Build history of the part. All positions in model axes, mm. Face numbers are marked on the shaded views. A direction names the side the tool comes from. Round coordinates to 2 decimals unless told otherwise and drop trailing zeros. Write each loop counter-clockwise with the first axis right and the second up, starting at its lowest first coordinate (ties: lowest second). Pieces come first, ordered by that corner, then holes.
1) Saw through at C-C (y = 7). Write the cut outline in (x, z), plus the area to 3 significant figures.
2) Which spindle directions (+Z, -Z, +X, -X, +Y, -Y) get a long thin tool onto all of the face, cutting with end or side? Do the marked faces 4, 5 and 6. Say none if no direction does.
3) Pull direction X, two halves, no side cores. Call the marked faces 1, 2 and 3: +X half, -X half, draft (parallel to the pull), parting line (faces both ways), or undercut.
4) Saw through at B-B (z = 2.5). Write the cut outline in (x, y), plus the area to 3 significant figures.
5) Saw through at A-A (y = -44). Write the cut outline in (x, z), plus the area to 3 significant figures.
6) Wall check: probe 1 along Z at (x, y) = (-31, -19.5); probe 2 along Y at (x, z) = (43, 16.5); probe 3 along Y at (x, z) = (-1, -1). Give the ranges that are in metal, low to high.
7) Flat gauge pins, fed straight in: pin 1 (5 mm diameter, centred on y = -24.5, z = 17, fed in from +X); pin 2 (4 mm diameter, centred on x = 3.5, y = 0.5, fed in from -Z); pin 3 (6 mm diameter, centred on x = -20.5, y = 0, fed in from +Z). Where does each tip first touch, or does it go through?
8) Saw through at D-D (x = 11). Write the cut outline in (y, z).
from build123d import *

# Parameters (mm, degrees)
EXTRUDE_1_DEPTH = 20
EXTRUDE_2_DEPTH = 25


with BuildPart() as part:
    # 草图3 → 凸台-拉伸1 (new body)
    with BuildSketch(Plane.XY):
        Polygon((0, -15), (0, 0), (-50, 0), (-50, -15), (-40, -15), (-16.127693207, -58.93305098), (-16.127693207, -15), align=None)
        Polygon((50, -15), (50, 0), (0, 0), (0, -15), (16.127693207, -15), (16.127693207, -58.93305098), (40, -15), align=None)
    extrude(amount=EXTRUDE_1_DEPTH)

    # 草图4 → 凸台-拉伸2 (add)
    with BuildSketch(Plane(origin=(0, 0, 0), x_dir=(1, 0, 0), z_dir=(0, 1, 0))):
        with BuildLine():
            Line((17.320508076, -20), (0, -20))
            Line((0, -20), (-17.320508076, -20))
            ThreePointArc((-17.320508076, -20), (0, -30), (17.320508076, -20))
        make_face()
        with BuildLine():
            Line((17.320508076, 0), (0, 0))
            Line((0, 0), (0, -20))
            Line((0, -20), (17.320508076, -20))
            ThreePointArc((17.320508076, -20), (19.318516526, -15.176380902), (20, -10))
            ThreePointArc((20, -10), (19.318516526, -4.823619098), (17.320508076, 0))
        make_face()
        with BuildLine():
            Line((0, -20), (0, 0))
            Line((0, 0), (-17.320508076, 0))
            ThreePointArc((-17.320508076, 0), (-20, -10), (-17.320508076, -20))
            Line((-17.320508076, -20), (0, -20))
        make_face()
        with BuildLine():
            Line((-17.320508076, 0), (0, 0))
            Line((0, 0), (17.320508076, 0))
            ThreePointArc((17.320508076, 0), (0, 10), (-17.320508076, 0))
        make_face()
    extrude(amount=EXTRUDE_2_DEPTH)


solid = part.part
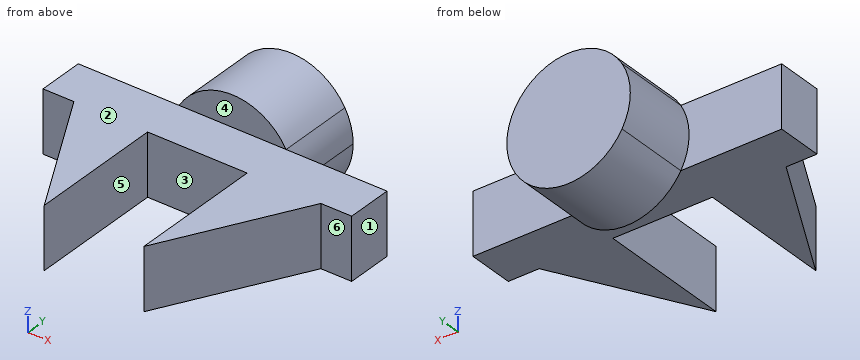
Evaluation:
1. outline: circle Ø40 at (0, 10)
1. area: 1,260 mm2
2. face 4: +Z, +X, -X, -Y
2. face 5: +Z, -Z, -Y
2. face 6: +Z, -Z, +X, -Y
3. face 1: +X half
3. face 2: draft
3. face 3: undercut
4. outline: (-50, -15) - (-40, -15) - (-16.13, -58.93) - (-16.13, -15) - (16.13, -15) - (16.13, -58.93) - (40, -15) - (50, -15) - (50, 0) - (18.54, 0) - (18.54, 25) - (-18.54, 25) - (-18.54, 0) - (-50, 0) - close
4. area: 3,480 mm2
5. outline: (-24.24, 0) - (-16.13, 0) - (-16.13, 20) - (-24.24, 20) - close; (16.13, 0) - (24.24, 0) - (24.24, 20) - (16.13, 20) - close
5. area: 325 mm2
6. probe 1: z = 0 to 20
6. probe 2: y = -15 to 0
6. probe 3: y = 0 to 25
7. pin 1: stops at x = 36.2
7. pin 2: stops at z = -9.94
7. pin 3: stops at z = 20
8. outline: (-15, 0) - (0, 0) - (0, -6.7) - (25, -6.7) - (25, 26.7) - (0, 26.7) - (0, 20) - (-15, 20) - close
